For this review, take the finished solid that the model builds, in its own axes (mm). Face numbers are marked on the shaded views. A direction names the side the tool comes from. Coordinates: 2 decimals unless noted, no trailing zeros. Order: outer loops, then holes, each group sorted by start corner. A loop starts at its lowest first (then second) coordinate and runs counter-clockwise, first axis right, second up. Notation, with made-up numbers: (22.5, -6) -> (70.5, -6) arc R17 cw to (70.5, 9) -> close; hole circle Ø2 at (50, 6). An arc over 180 degrees is marked (long way). Answer as a JSON object with one key per item and string values. Group by question number.
1) Wall thickness on L1, parallel to X at y = 52.3, z = -15; L2, parallel to Z at x = 7, y = 31; L3, parallel to Y at x = 14.25, z = -8: over which ranges is each line inside the solid? List them lowest first.
2) For pin 1 (10 mm diameter, centred on x = 13, y = 58, fed in from -Z); pin 2 (1.5 mm diameter, centred on x = 11, z = -3, fed in from +Y); pin 3 (10 mm diameter, centred on y = 33.5, z = -7.5, fed in from -X); pin 4 (6 mm diameter, centred on x = 15.5, z = -4.5, fed in from -Y), all flat-tipped, find the tip position at first contact; note any pin that passes through.
3) Add section C-C, the plane y = 33. Write out the cut boundary in (x, z).
4) Draft analysis for pull direction Z (two halves, no side actions). For the marked faces 3, 4 and 5, state which applies: +Z half, -Z half, draft (parallel to the pull), parting line (faces both ways), or undercut.
5) Machinability: for the marked faces 1 and 2, which of the approach directions +Z, -Z, +X, -X, +Y, -Y give a long, thin tool a straight path to every point of the face, cutting with its end or side? Answer none if there is none.
6) Add section A-A, the plane x = 9. Write out the cut boundary in (y, z).
7) Add section B-B, the plane z = -16. Write out the cut boundary in (x, y), then the cut area to 3 significant figures.
8) Add section D-D, the plane z = -6. Write out the cut boundary in (x, y).
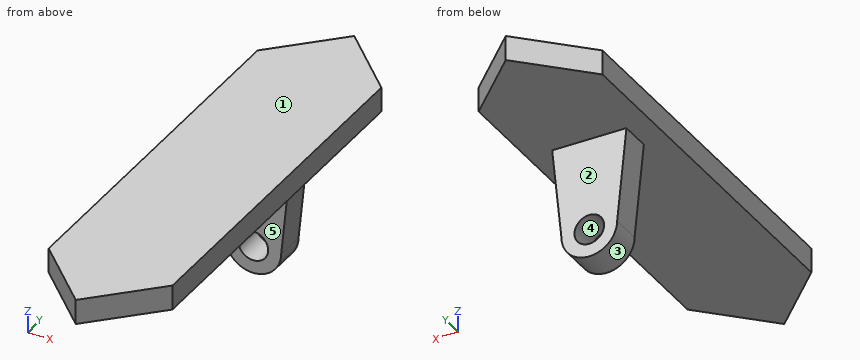
from build123d import *

# Parameters (mm, degrees)
EXTRUDE_1_DEPTH     = 4
SKETCH_2_W          = 12
SKETCH_2_H          = 5
EXTRUDE_2_DEPTH     = 20
SKETCH_6_R          = 2.4
CUT_EXTRUDE_5_DEPTH = 21


with BuildPart() as part:
    # 草图1 → 凸台-拉伸1 (new body)
    with BuildSketch(Plane.XY):
        Polygon((0.147281285, 10), (0.147281285, 70), (10.147281285, 80), (20.147281285, 70), (20.147281285, 10), (10.147281285, 0), align=None)
    extrude(amount=EXTRUDE_1_DEPTH)

    # 草图2 → 凸台-拉伸2 (add)
    with BuildSketch(Plane(origin=(0, 0, 0), x_dir=(-1, 0, 0), z_dir=(0, 0, -1))):
        with Locations((-10.147281285, 53.5)):
            Rectangle(SKETCH_2_W, SKETCH_2_H)
    extrude(amount=EXTRUDE_2_DEPTH)

    # 草图6 → 切除-拉伸5 (cut)
    with BuildSketch(Plane.XZ.offset(-51)):
        with Locations(Location((10.147281285, -15, 0), (0, 0, 270))):
            Circle(SKETCH_6_R)
        with BuildLine():
            ThreePointArc((14.647281285, -15), (10.147281285, -19.5), (5.647281285, -15))
            Line((5.647281285, -15), (4.147281285, 0))
            Line((4.147281285, 0), (4.147281285, -20))
            Line((4.147281285, -20), (16.147281285, -20))
            Line((16.147281285, -20), (16.147281285, 0))
            Line((16.147281285, 0), (14.647281285, -15))
        make_face()
    extrude(amount=-CUT_EXTRUDE_5_DEPTH, mode=Mode.SUBTRACT)


solid = part.part
Output values:
{
 "1": {"L1": "x = 5.65 to 7.75, 12.55 to 14.65", "L2": "z = 0 to 4", "L3": "y = 51 to 56"},
 "2": {"pin 1": "stops at z = -19.5", "pin 2": "stops at y = 56", "pin 3": "passes through", "pin 4": "stops at y = 51"},
 "3": {"outline": "(0.15, 0) -> (20.15, 0) -> (20.15, 4) -> (0.15, 4) -> close"},
 "4": {"face 3": "-Z half", "face 4": "undercut", "face 5": "draft"},
 "5": {"face 1": "+Z, +X, -X, +Y, -Y", "face 2": "-Z, +X, -X, +Y"},
 "6": {"outline": "(1.15, 0) -> (51, 0) -> (51, -12.89) -> (56, -12.89) -> (56, 0) -> (78.85, 0) -> (78.85, 4) -> (1.15, 4) -> close; (51, -19.35) -> (56, -19.35) -> (56, -17.11) -> (51, -17.11) -> close"},
 "7": {"outline": "(5.76, 51) -> (7.97, 51) -> (7.97, 56) -> (5.76, 56) -> close; (12.33, 51) -> (14.53, 51) -> (14.53, 56) -> (12.33, 56) -> close", "area": "22.1 mm²"},
 "8": {"outline": "(4.75, 51) -> (15.55, 51) -> (15.55, 56) -> (4.75, 56) -> close"}
}
